Could you check a few things on this model? Use its own coordinates, in mm. Face numbers are marked on the shaded views. Give positions to 0.01 mm unless a question says otherwise; leave off trailing zeros. Loops run counter-clockwise (first coordinate to the right, second up) from the corner with the lowest first, then second, coordinate; pieces in that order, holes last.
1. Imagine slicing it at B-B (z = 0). List the corners of the cut face in (x, y) for me (3 decimals), plus the area to 3 significant figures.
2. I need wall thicknesses on line 1 along Z through (x, y) = (0, 1.65); line 2 along X through (y, z) = (0.6, -5.5); line 3 along X through (y, z) = (0.25, -1.5). Which ranges of each line are inside material? Lowest first, please.
3. Thinking about a two-plate mould opening in X: for the marked faces 1, 2 and 3, which applies, +X half, -X half, draft (parallel to the pull), parting line (faces both ways), or undercut?
4. Imagine slicing it at A-A (x = 0). List the corners of the cut face in (y, z) for me (3 decimals).
5. Imagine slicing it at C-C (y = 2.35). List the corners of the cut face in (x, z) for me, plus the area to 3 significant figures.
6. For P1, Ø3, axis at x = 5.57, z = 5.57, coming from the +Y side (3 decimals), with a flat end and sliding along its axis, tell me the tip position at first contact or that it passes through.
```python
from build123d import *

# Parameters (mm, degrees)
SKETCH1_W           = 17.526
SKETCH1_H           = 17.526
SKETCH1_R           = 1
SKETCH1_R_2         = 5
BOSS_EXTRUDE1_DEPTH = 3.175


with BuildPart() as part:
    # Sketch1 → Boss-Extrude1 (new body)
    with BuildSketch(Plane(origin=(0, 0, 0), x_dir=(1, 0, 0), z_dir=(0, 1, 0))):
        Rectangle(SKETCH1_W, SKETCH1_H)
        with Locations((-5.567758795, 5.567758795)):
            Circle(SKETCH1_R, mode=Mode.SUBTRACT)
        with Locations((5.567758795, 5.567758795)):
            Circle(SKETCH1_R, mode=Mode.SUBTRACT)
        with Locations((5.567758795, -5.567758795)):
            Circle(SKETCH1_R, mode=Mode.SUBTRACT)
        with Locations((-5.567758795, -5.567758795)):
            Circle(SKETCH1_R, mode=Mode.SUBTRACT)
        Circle(SKETCH1_R_2, mode=Mode.SUBTRACT)
    extrude(amount=BOSS_EXTRUDE1_DEPTH)


solid = part.part
```
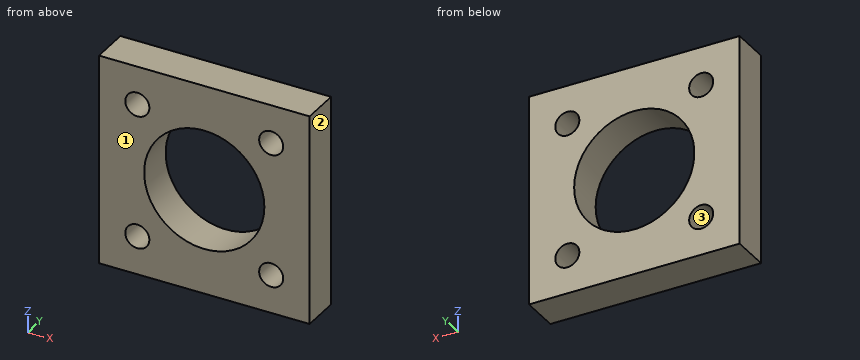
Derived:
1. outline: (-8.763, 0) - (-5, 0) - (-5, 3.175) - (-8.763, 3.175) - close; (5, 0) - (8.763, 0) - (8.763, 3.175) - (5, 3.175) - close
1. area: 23.9 mm2
2. line 1: z = -8.76 to -5, 5 to 8.76
2. line 2: x = -8.76 to -6.57, -4.57 to 4.57, 6.57 to 8.76
2. line 3: x = -8.76 to -4.77, 4.77 to 8.76
3. face 1: draft
3. face 2: +X half
3. face 3: undercut
4. outline: (0, -8.763) - (3.175, -8.763) - (3.175, -5) - (0, -5) - close; (0, 5) - (3.175, 5) - (3.175, 8.763) - (0, 8.763) - close
5. outline: (-8.76, -8.76) - (8.76, -8.76) - (8.76, 8.76) - (-8.76, 8.76) - close; hole circle Ø2 at (-5.57, -5.57); hole circle Ø2 at (-5.57, 5.57); hole circle Ø10 at (0, 0); hole circle Ø2 at (5.57, -5.57); hole circle Ø2 at (5.57, 5.57)
5. area: 216 mm2
6. P1: stops at y = 3.175
